Work out the finished part from the listing and answer in its coordinate system (mm). A direction names the side the tool comes from. Give positions to 0.01 mm unless a question says otherwise; leave off trailing zeros. Loops run counter-clockwise (first coordinate to the right, second up) from the corner with the lowest first, then second, coordinate; pieces in that order, holes last. Notation, with made-up numbers: M -1,43 L 40,43 A23 ccw 40,81 Z; hole C 40.5,39.25 d9. An arc over 180 degrees is marked long. Answer in a Markdown table with one row per item. Add a question column.
from build123d import *

# Parameters (mm, degrees)
SKETCH1_W           = 107
SKETCH1_H           = 87.7
BOSS_EXTRUDE1_DEPTH = 13.85
SKETCH2_W           = 102.38
SKETCH2_H           = 83.08
CUT_EXTRUDE1_DEPTH  = 7.9
SKETCH4_R           = 2.5
SKETCH4_R_2         = 1.2
BOSS_EXTRUDE2_DEPTH = 6.2
SKETCH7_W           = 11.25
SKETCH7_H           = 4.8
BOSS_EXTRUDE3_DEPTH = 1.7
BOSS_EXTRUDE4_DEPTH = 3.15
SKETCH3_W           = 23.5
SKETCH3_H           = 11.494748732
BOSS_EXTRUDE5_DEPTH = 4
SKETCH9_W           = 7.388623973
SKETCH9_H           = 2
CUT_EXTRUDE2_DEPTH  = 91.572539989
SKETCH10_W          = 47
SKETCH10_H          = 5.747374366
CUT_EXTRUDE4_DEPTH  = 72.670321612
CHAMFER1_SIZE       = 2
BOSS_EXTRUDE7_DEPTH = 1.5


with BuildPart() as part:
    # Sketch1 → Boss-Extrude1 (new body)
    with BuildSketch(Plane(origin=(0, 0, 0), x_dir=(1, 0, 0), z_dir=(0, 1, 0))):
        Rectangle(SKETCH1_W, SKETCH1_H)
    extrude(amount=BOSS_EXTRUDE1_DEPTH)

    # Sketch2 → Cut-Extrude1 (cut)
    with BuildSketch(Plane(origin=(0, 13.85, 0), x_dir=(1, 0, 0), z_dir=(0, 1, 0))):
        Rectangle(SKETCH2_W, SKETCH2_H)
    extrude(amount=-CUT_EXTRUDE1_DEPTH, mode=Mode.SUBTRACT)

    # Sketch4 → Boss-Extrude2 (add)
    # profile 1 of 2: a face of its own
    with BuildSketch(Plane(origin=(0, 5.95, 0), x_dir=(1, 0, 0), z_dir=(0, 1, 0))):
        with Locations(Location((-42.5, -25, 0), (0, 0, 90))):
            Circle(SKETCH4_R)
        with Locations(Location((-42.5, -25, 0), (0, 0, 90))):
            Circle(SKETCH4_R_2, mode=Mode.SUBTRACT)
    # profile 2 of 2: a face of its own
    with BuildSketch(Plane(origin=(0, 5.95, 0), x_dir=(1, 0, 0), z_dir=(0, 1, 0))):
        with Locations(Location((42.5, 25, 0), (0, 0, 90))):
            Circle(SKETCH4_R)
        with Locations(Location((42.5, 25, 0), (0, 0, 90))):
            Circle(SKETCH4_R_2, mode=Mode.SUBTRACT)
    extrude(amount=BOSS_EXTRUDE2_DEPTH)

    # Sketch7 → Boss-Extrude3 (add)
    with BuildSketch(Plane(origin=(-51.19, 0, 0), x_dir=(0, 0, -1), z_dir=(1, 0, 0))):
        with Locations((0, 8.35)):
            Rectangle(SKETCH7_W, SKETCH7_H)
    boss_extrude3 = extrude(amount=BOSS_EXTRUDE3_DEPTH)

    # Sketch8 → Boss-Extrude4 (add, symmetric)
    with BuildSketch(Plane.XY):
        Polygon((-49.49, 10.75), (-49.49, 18.75), (-50.99, 18.75), (-51.99, 16.75), (-51.19, 16.75), (-51.19, 10.75), align=None)
    boss_extrude4 = extrude(amount=BOSS_EXTRUDE4_DEPTH, both=True)

    # Sketch3 → Boss-Extrude5 (add)
    with BuildSketch(Plane.XZ):
        with Locations((-11.75, 8.992625634)):
            Rectangle(SKETCH3_W, SKETCH3_H)
        with Locations((11.75, 8.992625634)):
            Rectangle(SKETCH3_W, SKETCH3_H)
    extrude(amount=BOSS_EXTRUDE5_DEPTH)

    # Sketch9 → Cut-Extrude2 (cut, through all)
    with BuildSketch(Plane.ZY.offset(23.5)):
        with Locations((6.939563255, -1)):
            Rectangle(SKETCH9_W, SKETCH9_H)
    extrude(amount=-CUT_EXTRUDE2_DEPTH, mode=Mode.SUBTRACT)

    # Sketch10 → Cut-Extrude4 (cut, through all)
    with BuildSketch(Plane.XZ):
        with Locations((0, 6.118938451)):
            Rectangle(SKETCH10_W, SKETCH10_H)
    extrude(amount=-CUT_EXTRUDE4_DEPTH, mode=Mode.SUBTRACT)

    # Chamfer1
    chamfer1_edges = [part.edges().sort_by_distance(p)[0] for p in [
        (0, -2, 3.245251268),
    ]]
    chamfer(chamfer1_edges, length=CHAMFER1_SIZE - 0.0001)  # a hair under: the kernel refuses the full size

    # Mirror1: Boss-Extrude3, Boss-Extrude4 across plane
    add(boss_extrude3.mirror(Plane(origin=(0, 0, 0), x_dir=(0, 0, 1), z_dir=(1, 0, 0))))
    add(boss_extrude4.mirror(Plane(origin=(0, 0, 0), x_dir=(0, 0, 1), z_dir=(1, 0, 0))))

    # Sketch14 → Boss-Extrude7 (add)
    with BuildSketch(Plane.XZ):
        Polygon((-41.618061396, -23.418064695), (-46.893526608, -23.418064695), (-46.893526608, 0), (-35.18449426, 0), (-35.18449426, 14.74), (-23.5, 14.74), (-23.5, 10.633875241), (-29.707757231, 10.633875241), (-29.707757231, -4.071607842), (-41.618061396, -4.071607842), align=None)
    boss_extrude7 = extrude(amount=BOSS_EXTRUDE7_DEPTH)

    # Mirror2: Boss-Extrude7 across plane
    add(boss_extrude7.mirror(Plane(origin=(0, 0, 0), x_dir=(0, 0, 1), z_dir=(1, 0, 0))))


solid = part.part
(1) Which of the six approach directions +Z, -Z, +X, -X, +Y, -Y give full straight-line access (tool end or side, diameter ignored) to faces 4 (the face through (-23.5, -3, 10)), 5 (the face through (0, -4, 9)), 6 (the face through (-53.5, 7, 1)), 7 (the face through (38, -1.5, -3)), 8 (the face through (-23.5, 3, 6))?
(2) Section D-D, the plane x = 28 is taken. Determine the outline of the cut face in (y, z), and give its area (3 significant figures).
(3) The mould has two halves that part along Z. Classify faces 1 (the face through (-1, 7, 43.85)), 2 (the face through (-50, 15, 3.15)), 3 (the face through (51.19, 15, 0)): pulls with the +Z half, pulls with the -Z half, needs draft (parallel to the pull), parting line crosses it, or undercut.
(4) Section A-A, the plane y = 7.25 is taken. Determine the outline of the cut face in (x, z) (3 decimals), and give its area (3 significant figures).
(5) Consider line 1 along Z through (x, y) = (-42.5, 10.5); line 2 along X through (y, z) = (7.75, 25); line 3 along Z through (x, y) = (42.5, 8.25). Determine where each line is inside the solid, lowest interval first. Write a range as from..to.
(6) Each of these flat-tipped pins is pushed along its axis until it touches: P1, Ø1.9, axis at x = 50.5, z = -4.5, coming from the +Y side; P2, Ø1.4, axis at x = -50, z = -4, coming from the +Y side; P3, Ø1.9, axis at x = -42, z = 25, coming from the +Y side. Where does it stop, or does it pass through?
(7) Section B-B, the plane z = 25 is taken. Determine the outline of the cut face in (x, y), and give its area (3 significant figures).
(8) Section C-C, the plane y = 2.25 is taken. Determine the outline of the cut face in (x, z).
Numbers:
| question | item | result |
|---|---|---|
| 1 | face 4 | +Z, -Z, -X, -Y |
| 1 | face 5 | +Z, -Z, +X, -X, -Y |
| 1 | face 6 | +Z, -Z, -X, +Y, -Y |
| 1 | face 7 | +Z, -Z, +X, -Y |
| 1 | face 8 | +Y |
| 2 | outline | M -1.5,10.63 L 0,10.63 L 0,-43.85 L 13.85,-43.85 L 13.85,-41.54 L 5.95,-41.54 L 5.95,41.54 L 13.85,41.54 L 13.85,43.85 L 0,43.85 L 0,14.74 L -1.5,14.74 Z |
| 2 | area | 564 mm² |
| 3 | face 1 | pulls with the +Z half |
| 3 | face 2 | undercut |
| 3 | face 3 | needs draft |
| 4 | outline | M -53.5,-43.85 L 53.5,-43.85 L 53.5,43.85 L -53.5,43.85 Z; C -42.5,25 d5; C 42.5,-25 d5; hole M -51.19,-41.54 L 51.19,-41.54 L 51.19,-5.625 L 49.49,-5.625 L 49.49,5.625 L 51.19,5.625 L 51.19,41.54 L -51.19,41.54 L -51.19,5.625 L -49.49,5.625 L -49.49,-5.625 L -51.19,-5.625 Z; hole C -42.5,25 d2.4; hole C 42.5,-25 d2.4 |
| 4 | area | 947 mm² |
| 5 | line 1 | z = -43.85..-41.54, 22.5..23.8, 26.2..27.5, 41.54..43.85 |
| 5 | line 2 | x = -53.5..-51.19, -45..-43.7, -41.3..-40, 51.19..53.5 |
| 5 | line 3 | z = -43.85..-41.54, -27.5..-26.2, -23.8..-22.5, 41.54..43.85 |
| 6 | P1 | stops at y = 13.85 |
| 6 | P2 | stops at y = 10.75 |
| 6 | P3 | stops at y = 12.15 |
| 7 | outline | M -53.5,0 L 53.5,0 L 53.5,13.85 L 51.19,13.85 L 51.19,5.95 L -40,5.95 L -40,12.15 L -41.3,12.15 L -41.3,5.95 L -43.7,5.95 L -43.7,12.15 L -45,12.15 L -45,5.95 L -51.19,5.95 L -51.19,13.85 L -53.5,13.85 Z |
| 7 | area | 689 mm² |
| 8 | outline | M -53.5,-43.85 L 53.5,-43.85 L 53.5,43.85 L -53.5,43.85 Z; hole M -23.5,3.25 L 23.5,3.25 L 23.5,8.99 L -23.5,8.99 Z |
